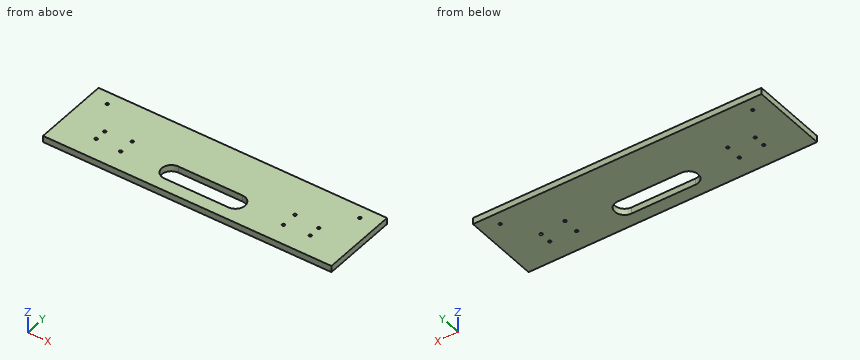
from build123d import *

# Parameters (mm, degrees)
SCHIZZO1_W                   = 450
SCHIZZO1_H                   = 120
ESTRUSIONE_ESTRUSIONE1_DEPTH = 10
TAGLIO_ESTRUSIONE1_DEPTH     = 10
SCHIZZO3_R                   = 2.25
TAGLIO_ESTRUSIONE2_DEPTH     = 10
SCHIZZO4_R                   = 2.25
TAGLIO_ESTRUSIONE3_DEPTH     = 10


with BuildPart() as part:
    # Schizzo1 → Estrusione-Estrusione1 (new body)
    with BuildSketch(Plane.XY):
        Rectangle(SCHIZZO1_W, SCHIZZO1_H)
    extrude(amount=ESTRUSIONE_ESTRUSIONE1_DEPTH)

    # Schizzo2 → Taglio-Estrusione1 (cut)
    with BuildSketch(Plane(origin=(0, 0, 0), x_dir=(-1, 0, 0), z_dir=(0, 0, -1))):
        with BuildLine():
            Line((-50, -10), (50, -10))
            ThreePointArc((50, -10), (65, -25), (50, -40))
            Line((50, -40), (-50, -40))
            ThreePointArc((-50, -40), (-65, -25), (-50, -10))
        make_face()
    extrude(amount=-TAGLIO_ESTRUSIONE1_DEPTH, mode=Mode.SUBTRACT)

    # Schizzo3 → Taglio-Estrusione2 (cut)
    with BuildSketch(Plane.XY.offset(10)):
        with Locations((-167, -7)):
            Circle(SCHIZZO3_R)
        with Locations((-167, -25.5)):
            Circle(SCHIZZO3_R)
        with Locations((167, -7)):
            Circle(SCHIZZO3_R)
        with Locations((167, -25.5)):
            Circle(SCHIZZO3_R)
        with Locations((197, 40)):
            Circle(SCHIZZO3_R)
        with Locations((-197, 40)):
            Circle(SCHIZZO3_R)
    extrude(amount=-TAGLIO_ESTRUSIONE2_DEPTH, mode=Mode.SUBTRACT)

    # Schizzo4 → Taglio-Estrusione3 (cut)
    with BuildSketch(Plane(origin=(0, 0, 0), x_dir=(-1, 0, 0), z_dir=(0, 0, -1))):
        with Locations((-127, -3)):
            Circle(SCHIZZO4_R)
        with Locations((-127, -28)):
            Circle(SCHIZZO4_R)
        with Locations((127, -28)):
            Circle(SCHIZZO4_R)
        with Locations((127, -3)):
            Circle(SCHIZZO4_R)
    extrude(amount=-TAGLIO_ESTRUSIONE3_DEPTH, mode=Mode.SUBTRACT)


solid = part.part
Geometry: final body of the model. Coordinates: model frame, mm. Give positions to 0.01 mm unless a question says otherwise; leave off trailing zeros. Order: outer loops, then holes, each group sorted by start corner. A loop starts at its lowest first (then second) coordinate and runs counter-clockwise, first axis right, second up. Notation, with made-up numbers: (-27, -32.75) -> (25, -32.75) arc R21 ccw to (25, -5.75) -> close; hole circle Ø1 at (-16.5, 15). An arc over 180 degrees is marked (long way). Put each result on its own line as item: value.
Q1. Section A-A, the plane x = 30. Return loops of the section in (y, z), then the cut area to 3 significant figures.
Here are the results:
outline: (-60, 0) -> (-40, 0) -> (-40, 10) -> (-60, 10) -> close; (-10, 0) -> (60, 0) -> (60, 10) -> (-10, 10) -> close
area: 900 mm^2
Q2. Section B-B, the plane z = 4.75. Count the separate pieces of the cut face and the enclosed holes in it, then the cut area to 3 significant figures.
Here are the results:
separate pieces: 1
enclosed holes: 11
area: 50,100 mm^2
Q3. Pin query (flat end, axial travel): pin 1 (2.5 mm diameter, centred on x = 197, y = 40, fed in from +Z). Return the tip coordinate at first contact, or that it passes through.
Here are the results:
pin 1: passes through
Q4. Material intervals for L1, parallel to Y at x = 127, z = 4.75; L2, parallel to Y at x = -167, z = 4.25; L3, parallel to Y at x = -197, z = 7.75, sorted ascending.
Here are the results:
L1: y = -60 to -30.25, -25.75 to -5.25, -0.75 to 60
L2: y = -60 to -27.75, -23.25 to -9.25, -4.75 to 60
L3: y = -60 to 37.75, 42.25 to 60
